from build123d import *

# Parameters (mm, degrees)
BOSS_EXTRUDE1_DEPTH = 6
BOSS_EXTRUDE2_DEPTH = 6
SKETCH2_R           = 2
CUT_EXTRUDE1_DEPTH  = 7


with BuildPart() as part:
    # Sketch1 → Boss-Extrude1 (new body)
    with BuildSketch(Plane(origin=(0, 0, 0), x_dir=(1, 0, 0), z_dir=(0, 1, 0))):
        with BuildLine():
            Line((5, 33), (5, 0))
            Line((5, 0), (5, -17))
            ThreePointArc((5, -17), (-0.5, -22.5), (-6, -17))
            Line((-6, -17), (-6, 0))
            Line((-6, 0), (-6, 33))
            ThreePointArc((-6, 33), (-0.5, 38.5), (5, 33))
        make_face()
    extrude(amount=BOSS_EXTRUDE1_DEPTH)

    # Sketch4 → Boss-Extrude2 (add)
    with BuildSketch(Plane(origin=(0, 6, 0), x_dir=(1, 0, 0), z_dir=(0, 1, 0))):
        with BuildLine():
            Line((0, 18.405260039), (0, -22.486700485))
            ThreePointArc((0, -22.486700485), (0.153171428, -22.74508915), (0.315483204, -22.99783621))
            ThreePointArc((0.315483204, -22.99783621), (0.859997468, -22.98391621), (1.404029403, -22.957105685))
            ThreePointArc((1.404029403, -22.957105685), (2.272765962, -20.722115477), (2.474630782, -18.332735843))
            ThreePointArc((2.474630782, -18.332735843), (3.439178821, -18.176497188), (4.39413166, -17.969546682))
            ThreePointArc((4.39413166, -17.969546682), (5.454980724, -20.120007959), (7.080198393, -21.883116568))
            ThreePointArc((7.080198393, -21.883116568), (7.596418425, -21.709316597), (8.108378007, -21.52334096))
            ThreePointArc((8.108378007, -21.52334096), (8.279744109, -19.1315805), (7.76835863, -16.7888536))
            ThreePointArc((7.76835863, -16.7888536), (8.644002354, -16.355250664), (9.495529586, -15.876017098))
            ThreePointArc((9.495529586, -15.876017098), (11.143107691, -17.618248663), (13.215806885, -18.823985986))
            ThreePointArc((13.215806885, -18.823985986), (13.657864268, -18.505748935), (14.092261641, -18.177132938))
            ThreePointArc((14.092261641, -18.177132938), (13.551030657, -15.841120639), (12.371833724, -13.753208037))
            ThreePointArc((12.371833724, -13.753208037), (13.080768345, -13.080768345), (13.753208037, -12.371833724))
            ThreePointArc((13.753208037, -12.371833724), (15.841120639, -13.551030657), (18.177132938, -14.092261641))
            ThreePointArc((18.177132938, -14.092261641), (18.505748935, -13.657864268), (18.823985986, -13.215806885))
            ThreePointArc((18.823985986, -13.215806885), (17.618248663, -11.143107691), (15.876017098, -9.495529586))
            ThreePointArc((15.876017098, -9.495529586), (16.355250664, -8.644002354), (16.7888536, -7.76835863))
            ThreePointArc((16.7888536, -7.76835863), (19.1315805, -8.279744109), (21.52334096, -8.108378007))
            ThreePointArc((21.52334096, -8.108378007), (21.709316597, -7.596418425), (21.883116568, -7.080198393))
            ThreePointArc((21.883116568, -7.080198393), (20.120007959, -5.454980724), (17.969546682, -4.39413166))
            ThreePointArc((17.969546682, -4.39413166), (18.176497188, -3.439178821), (18.332735843, -2.474630782))
            ThreePointArc((18.332735843, -2.474630782), (20.722115477, -2.272765962), (22.957105685, -1.404029403))
            ThreePointArc((22.957105685, -1.404029403), (22.98391621, -0.859997468), (22.99783621, -0.315483204))
            ThreePointArc((22.99783621, -0.315483204), (20.834016252, 0.717845219), (18.466403185, 1.097704147))
            ThreePointArc((18.466403185, 1.097704147), (18.382682171, 2.071230843), (18.247674055, 3.038978872))
            ThreePointArc((18.247674055, 3.038978872), (20.471399556, 3.936157414), (22.351030824, 5.425073374))
            ThreePointArc((22.351030824, 5.425073374), (22.216294005, 5.952838037), (22.069097181, 6.477264053))
            ThreePointArc((22.069097181, 6.477264053), (19.696830773, 6.826887464), (17.322438727, 6.492004123))
            ThreePointArc((17.322438727, 6.492004123), (16.955485171, 7.397602558), (16.541226348, 8.282561916))
            ThreePointArc((16.541226348, 8.282561916), (18.401709947, 9.795335931), (19.758968788, 11.772134574))
            ThreePointArc((19.758968788, 11.772134574), (19.474656582, 12.23673776), (19.179422019, 12.694477974))
            ThreePointArc((19.179422019, 12.694477974), (16.809495442, 12.329330799), (14.63929957, 11.309461043))
            ThreePointArc((14.63929957, 11.309461043), (14.021718906, 12.066664821), (13.365018091, 12.790202986))
            ThreePointArc((13.365018091, 12.790202986), (14.696947654, 14.784155864), (15.411235665, 17.073189956))
            ThreePointArc((15.411235665, 17.073189956), (15.002610459, 17.433349632), (14.585571043, 17.783731818))
            ThreePointArc((14.585571043, 17.783731818), (12.428562673, 16.736258985), (10.655394403, 15.122022719))
            ThreePointArc((10.655394403, 15.122022719), (9.842061383, 15.663550962), (9.001269325, 16.161378393))
            ThreePointArc((9.001269325, 16.161378393), (9.686297066, 18.459338669), (9.694146621, 20.857217487))
            ThreePointArc((9.694146621, 20.857217487), (9.197516559, 21.080931885), (8.695728072, 21.292823047))
            ThreePointArc((8.695728072, 21.292823047), (6.913991789, 19.619372088), (5.689483487, 17.503810292))
            ThreePointArc((5.689483487, 17.503810292), (2.880227161, 18.178500725), (0, 18.405260039))
        make_face()
    extrude(amount=-BOSS_EXTRUDE2_DEPTH)

    # Sketch2 → Cut-Extrude1 (cut, through all)
    with BuildSketch(Plane(origin=(0, 6, 0), x_dir=(1, 0, 0), z_dir=(0, 1, 0))):
        Circle(SKETCH2_R)
        with Locations((0, 33)):
            Circle(SKETCH2_R)
        with BuildLine():
            Line((1.5, 17), (1.5, 13))
            ThreePointArc((1.5, 13), (0, 11.5), (-1.5, 13))
            Line((-1.5, 13), (-1.5, 17))
            ThreePointArc((-1.5, 17), (0, 18.5), (1.5, 17))
        make_face()
        with BuildLine():
            Line((-1.5, -17), (-1.5, -13))
            ThreePointArc((-1.5, -13), (0, -11.5), (1.5, -13))
            Line((1.5, -13), (1.5, -17))
            ThreePointArc((1.5, -17), (0, -18.5), (-1.5, -17))
        make_face()
    extrude(amount=-CUT_EXTRUDE1_DEPTH, mode=Mode.SUBTRACT)


solid = part.part
Work out the finished part from the listing and answer in its coordinate system (mm). A direction names the side the tool comes from. Round coordinates to 2 decimals unless told otherwise and drop trailing zeros. Write each loop counter-clockwise with the first axis right and the second up, starting at its lowest first coordinate (ties: lowest second). Pieces come first, ordered by that corner, then holes.
1) A tool of negligible diameter and unlimited length cuts with its end or side. For faces 1 (the cylindrical face through (8.632, 3.042, 16.362)), 2 (the cylindrical face through (20.148, 3.042, 5.474)), 3 (the cylindrical face through (22.984, 3.042, 0.868)), from which of +Z, -Z, +X, -X, +Y, -Y can it reach the whole face along a straight path? Write none if from no direction.
2) The mould has two halves that part along Z. Classify faces 4 (the flat face through (-6, 3, -8)), 5 (the cylindrical face through (0, 3, -18.5)), 6 (the cylindrical face through (12.456, 3.042, -16.755)): pulls with the +Z half, pulls with the -Z half, needs draft (parallel to the pull), parting line crosses it, or undercut.
3) A cutting plane is placed at C-C (z = 5). Give the vertices of the cut face in (x, y).
4) A cutting plane is placed at A-A (y = 4.45). Give the number of separate pieces and of enclosed holes in the cut face, plus the area to 3 significant figures.
5) A cutting plane is placed at B-B (x = -3.5). Give the vertices of the cut face in (y, z).
6) Straight lines are drawn through the part: line 1 (X direction, y = 3.65, z = -33); line 2 (X direction, y = 2.9, z = -17); line 3 (Z direction, x = 0, y = 4). For each, find the intervals that lie inside material, in ascending order.
7) Given pin 1 Ø1.5 at (x, y) = (8, 4.5) entering from +Z; pin 2 Ø1.2 at (y, z) = (4, -15) entering from +X; pin 3 Ø2 at (y, z) = (3, 14.5) entering from +X, each flat-ended and moving along its own axis, determine where each tip first touches the part or whether it passes through.
Completed:
1. face 1: +Y, -Y
1. face 2: +X, +Y, -Y
1. face 3: +Z, +X, +Y, -Y
2. face 4: needs draft
2. face 5: undercut
2. face 6: pulls with the -Z half
3. outline: (-6, 0) - (19.38, 0) - (19.38, 6) - (-6, 6) - close
4. separate pieces: 1
4. enclosed holes: 4
4. area: 1,050 mm2
5. outline: (0, -37.61) - (6, -37.61) - (6, 21.61) - (0, 21.61) - close
6. line 1: x = -6 to -2, 2 to 5
6. line 2: x = -6 to -1.5, 1.5 to 9.34, 12.84 to 15.4
6. line 3: z = -38.48 to -35, -31 to -18.5, -11.5 to -2, 2 to 11.5, 18.5 to 22.48
7. pin 1: stops at z = 21.83
7. pin 2: stops at x = 15.04
7. pin 3: stops at x = 18.62
